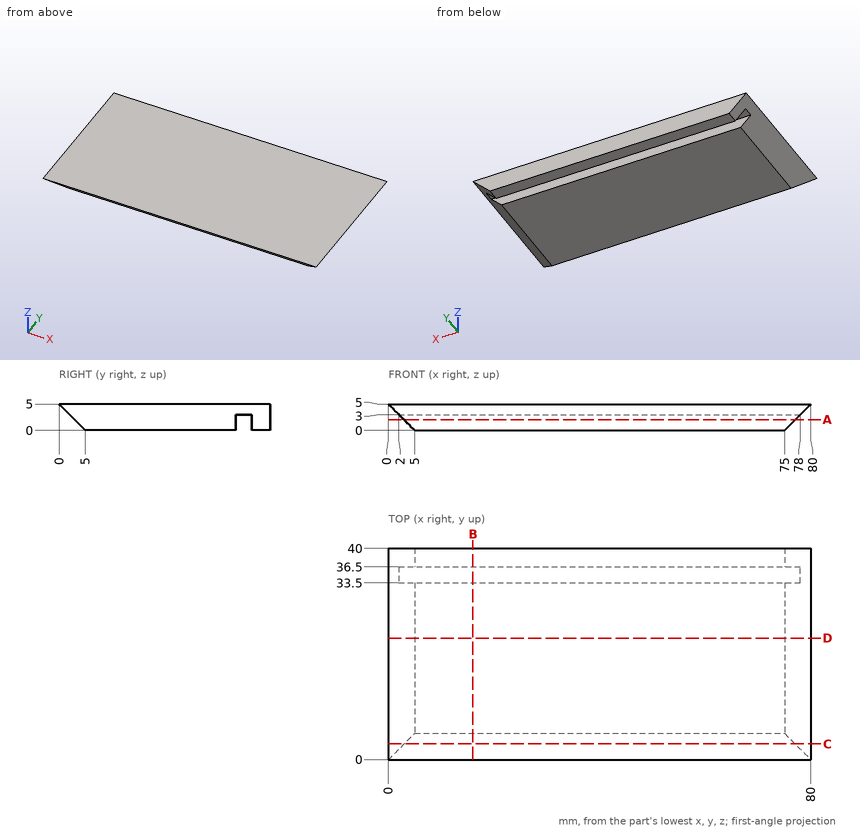
Could you check a few things on this drawing? It's one solid part, dimensions in mm from its lowest x, y, z. Give positions to 0.01 mm unless a question says otherwise; leave off trailing zeros. Order: outer loops, then holes, each group sorted by start corner. A loop starts at its lowest first (then second) coordinate and runs counter-clockwise, first axis right, second up. Notation, with made-up numbers: (28, -29.5) - (59, -29.5) arc R13 ccw to (59, -9.5) - close; hole circle Ø3 at (70.25, 35.5). An arc over 180 degrees is marked (long way). Answer as a JSON object with one key per item and string values. Group by question number.
Item 1: If we section it at B-B on x = 16: Please give me the cut outline in (y, z).
Item 2: If we section it at D-D on y = 23: Please give me the cut outline in (x, z).
Item 3: Please list where these lines run through material, in increasing order: probe 1 along Y at (x, z) = (56, 2.9); probe 2 along Z at (x, y) = (13.5, 2); probe 3 along Y at (x, z) = (74, 1.4).
Item 4: If we section it at A-A on z = 2.05: Please give me the cut outline in (x, y), and give its area (3 significant figures).
Item 5: If we section it at C-C on y = 3: Please give me the cut outline in (x, z), and give its area (3 significant figures).
Item 6: For P1, Ø2, axis at y = 4.5, z = 1.5, coming from the -X side; P2, Ø0.9, axis at x = 32.5, y = 35.5, coming from the -Z side; P3, Ø1.5, axis at y = 32, z = 3.5, coming from the +X side, each with a flat end and sliding along its axis, tell me the tip position at first contact or that it passes through.
Result set:
{
 "1": {"outline": "(0, 5) - (5, 0) - (33.5, 0) - (33.5, 3) - (36.5, 3) - (36.5, 0) - (40, 0) - (40, 5) - close"},
 "2": {"outline": "(0, 5) - (5, 0) - (75, 0) - (80, 5) - close"},
 "3": {"probe 1": "2.1 to 33.5, 36.5 to 40", "probe 2": "3 to 5", "probe 3": "3.6 to 33.5, 36.5 to 40"},
 "4": {"outline": "(2.95, 2.95) - (77.05, 2.95) - (77.05, 33.5) - (2.95, 33.5) - close; (2.95, 36.5) - (77.05, 36.5) - (77.05, 40) - (2.95, 40) - close", "area": "2,520 mm²"},
 "5": {"outline": "(0, 5) - (3, 2) - (77, 2) - (80, 5) - close", "area": "231 mm²"},
 "6": {"P1": "x = 2.5", "P2": "z = 3", "P3": "x = 79.25"}
}
